Work out the finished part from the listing and answer in its coordinate system (mm). A direction names the side the tool comes from. Coordinates: 2 decimals unless noted, no trailing zeros. Loops run counter-clockwise (first coordinate to the right, second up) from the corner with the lowest first, then second, coordinate; pieces in that order, holes last. Notation, with made-up numbers: (31.25, -38) - (35.25, -38) arc R17 ccw to (35.25, -27) - close; hole circle Ø5 at (-10, -17). An arc over 180 degrees is marked (long way). Write each question's results on one line, items separated by ' | '. Start each with the question number.
Item 1: Section A-A, the plane x = -2 is taken. Write down the section's boundary in (y, z).
Item 2: For a pull along Z with two mould halves and no side action, classify faces 1 (the face through (-69.695, -2, 38)), 2 (the face through (-67, -2, 41.002)), 3 (the face through (76, -2, 14.252)), 4 (the face through (-25.695, -2, 19)) as +Z half, -Z half, draft (parallel to the pull), parting line (faces both ways), or undercut.
Item 3: Each of these flat-tipped pins is pushed along its axis until it touches: pin 1 Ø1.5 at (y, z) = (-3.5, 40.5) entering from -X; pin 2 Ø1.6 at (y, z) = (0.5, -1.5) entering from -X; pin 3 Ø2.5 at (y, z) = (-3, -27.5) entering from +X; pin 4 Ø1.5 at (y, z) = (-2.5, -18) entering from -X. Where does it stop, or does it pass through?
Item 4: Consider probe 1 along X at (y, z) = (-1.75, 40); probe 2 along X at (y, z) = (-0.5, -3.5); probe 3 along X at (y, z) = (1, 14). Determine where each line is inside the solid, lowest interval first. Write a range as [from, to].
Item 5: A tool of negligible diameter and unlimited length cuts with its end or side. For faces 5 (the face through (-24, -2, 0.006)), 6 (the face through (-24, -2, -30.294)), 7 (the face through (27.75, -2, -3)), from which of +Z, -Z, +X, -X, +Y, -Y can it reach the whole face along a straight path? Write none if from no direction.
Item 6: Section B-B, the plane y = -2.5 is taken. Count the separate pieces of the cut face and the enclosed holes in it, plus the area to 4 significant figures.
from build123d import *

# Parameters (mm, degrees)
SKETCH_1_W          = 200
SKETCH_1_H          = 115
EXTRUDE_1_DEPTH     = 1.5
SKETCH_2_W          = 203
SKETCH_2_H          = 118
EXTRUDE_2_DEPTH     = 1.5
SKETCH_3_W          = 15
SKETCH_3_H          = 10
CUT_EXTRUDE_1_DEPTH = 11.5
FILLET_2_R          = 1
FILLET_3_R          = 1
SKETCH_4_W          = 8
SKETCH_4_H          = 1.5
EXTRUDE_3_DEPTH     = 5


with BuildPart() as part:
    # 草图1 → 凸台-拉伸1 (new body)
    with BuildSketch(Plane(origin=(0, 0, 0), x_dir=(1, 0, 0), z_dir=(0, 1, 0))):
        Rectangle(SKETCH_1_W, SKETCH_1_H)
    extrude(amount=EXTRUDE_1_DEPTH)

    # 草图2 → 凸台-拉伸2 (add)
    with BuildSketch(Plane(origin=(0, 1.5, 0), x_dir=(1, 0, 0), z_dir=(0, 1, 0))):
        Rectangle(SKETCH_2_W, SKETCH_2_H)
    extrude(amount=EXTRUDE_2_DEPTH)

    # 草图3 → 切除-拉伸1 (cut)
    with BuildSketch(Plane.XZ):
        with Locations((0, -47.14798892)):
            Rectangle(SKETCH_3_W, SKETCH_3_H)
    extrude(amount=-CUT_EXTRUDE_1_DEPTH, mode=Mode.SUBTRACT)

    # 圆角2
    fillet_2_edges = [part.edges().sort_by_distance(p)[0] for p in [
        (0, 3, -42.14798892),
        (-7.5, 3, -47.14798892),
        (0, 3, -52.14798892),
        (7.5, 3, -47.14798892),
        (7.5, 1.5, -42.14798892),
        (7.5, 1.5, -52.14798892),
        (-7.5, 1.5, -52.14798892),
        (-7.5, 1.5, -42.14798892),
        (7.5, 0, -47.14798892),
        (0, 0, -42.14798892),
        (-7.5, 0, -47.14798892),
        (0, 0, -52.14798892),
    ]]
    fillet(fillet_2_edges, radius=FILLET_2_R)

    # 圆角3
    fillet_3_edges = [part.edges().sort_by_distance(p)[0] for p in [
        (101.5, 3, 0),
        (0, 3, -59),
        (-101.5, 3, 0),
        (0, 3, 59),
    ]]
    fillet(fillet_3_edges, radius=FILLET_3_R)

    # 草图4 → 凸台-拉伸3 (add)
    with BuildSketch(Plane.XZ):
        Polygon((-64.695285942, 41.001921469), (-64.695285942, 42.501921469), (-71.195285942, 42.501921469), (-71.195285942, 36.001921469), (-69.695285942, 36.001921469), (-69.695285942, 41.001921469), align=None)
        Polygon((-21.25, -1.493976955), (-21.25, 0.006023045), (-27.75, 0.006023045), (-27.75, -6.493976955), (-26.25, -6.493976955), (-26.25, -1.493976955), align=None)
        Polygon((-32.195285942, 41.001921469), (-32.195285942, 42.501921469), (-25.695285942, 42.501921469), (-25.695285942, 36.001921469), (-27.195285942, 36.001921469), (-27.195285942, 41.001921469), align=None)
        Polygon((-25.695285942, 22.001921469), (-27.195285942, 22.001921469), (-27.195285942, 17.001921469), (-32.195285942, 17.001921469), (-32.195285942, 15.501921469), (-25.695285942, 15.501921469), align=None)
        Polygon((-71.195285942, 22.001921469), (-69.695285942, 22.001921469), (-69.695285942, 17.001921469), (-64.695285942, 17.001921469), (-64.695285942, 15.501921469), (-71.195285942, 15.501921469), align=None)
        Polygon((27.75, -6.493976955), (26.25, -6.493976955), (26.25, -1.493976955), (21.25, -1.493976955), (21.25, 0.006023045), (27.75, 0.006023045), align=None)
        Polygon((-26.25, -30.293976955), (-21.25, -30.293976955), (-21.25, -31.793976955), (-27.75, -31.793976955), (-27.75, -25.293976955), (-26.25, -25.293976955), align=None)
        Polygon((21.25, -30.293976955), (21.25, -31.793976955), (27.75, -31.793976955), (27.75, -25.293976955), (26.25, -25.293976955), (26.25, -30.293976955), align=None)
        with Locations((52.085748654, 44.501921469)):
            Rectangle(SKETCH_4_W, SKETCH_4_H)
        Polygon((25.335748654, 19.251921469), (23.835748654, 19.251921469), (23.835748654, 12.751921469), (30.335748654, 12.751921469), (30.335748654, 14.251921469), (25.335748654, 14.251921469), align=None)
        Polygon((73.835748654, 12.751921469), (73.835748654, 14.251921469), (78.835748654, 14.251921469), (78.835748654, 19.251921469), (80.335748654, 19.251921469), (80.335748654, 12.751921469), align=None)
    extrude(amount=EXTRUDE_3_DEPTH)


solid = part.part
Answer key:
1) outline: (0, -57.5) - (1.5, -57.5) - (1.5, -59) - (2, -59) arc R1 ccw to (3, -58) - (3, -53.15) arc R1 ccw to (2, -52.15) - (1, -52.15) arc R1 ccw to (0, -53.15) - close; (0, -41.15) arc R1 ccw to (1, -42.15) - (2, -42.15) arc R1 ccw to (3, -41.15) - (3, 58) arc R1 ccw to (2, 59) - (1.5, 59) - (1.5, 57.5) - (0, 57.5) - close
2) face 1: undercut | face 2: undercut | face 3: +Z half | face 4: draft
3) pin 1: stops at x = -71.2 | pin 2: stops at x = -100 | pin 3: stops at x = 27.75 | pin 4: passes through
4) probe 1: x = [-71.2, -69.7], [-27.2, -25.7] | probe 2: x = [-27.75, -26.25], [26.25, 27.75] | probe 3: x = [-100, 100]
5) face 5: +X, -X, -Y | face 6: -Y | face 7: -Z, +X, -Y
6) separate pieces: 11 | enclosed holes: 0 | area: 184.5 mm^2
